Here's the drawing with two shaded views (mm, measured from the low corner). I have some questions. A direction names the side the tool comes from. Coordinates: 2 decimals unless noted, no trailing zeros. Write each loop counter-clockwise with the first axis right and the second up, starting at its lowest first coordinate (ties: lowest second). Pieces come first, ordered by that corner, then holes. Notation, with made-up numbers: (65.25, 66.5) -> (95.25, 66.5) arc R11 cw to (95.25, 71.5) -> close; hole circle Ø8 at (-11, 5). An arc over 180 degrees is marked (long way). Put each result on its own line as item: value.
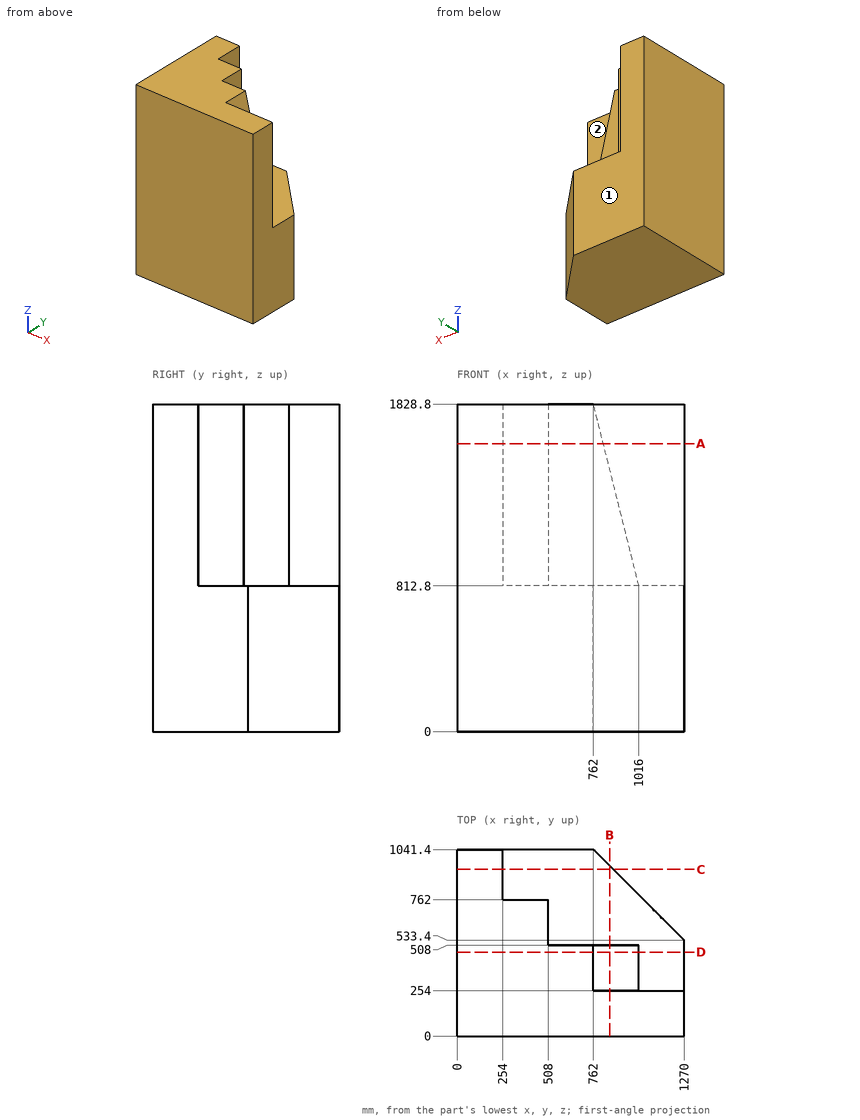
Item 1: Which directions (+Z, -Z, +X, -X, +Y, -Y) give clear straight access to the entire face, cutting with the end or side of a thin tool? Please do the marked faces 1 and 2.
Output:
face 1: +Z, -Z, +X, -X, +Y
face 2: +Z, +X, +Y
Item 2: Imagine slicing it at C-C on y = 930. Write out the boundary of the cut face in (x, z).
Output:
outline: (0, 0) -> (873.4, 0) -> (873.4, 812.8) -> (254, 812.8) -> (254, 1828.8) -> (0, 1828.8) -> close
Item 3: Imagine slicing it at D-D on y = 469. Write out the boundary of the cut face in (x, z), then the cut area to 3 significant figures.
Output:
outline: (0, 0) -> (1270, 0) -> (1270, 812.8) -> (1016, 812.8) -> (762, 1828.8) -> (0, 1828.8) -> close
area: 1,940,000 mm²
Item 4: Please list where these lines run through material, in increasing order: line 1 along X through (y, z) = (530, 1155.5); line 2 along X through (y, z) = (935.5, 972); line 3 along Z through (x, y) = (901, 548). Write a range as from..to.
Output:
line 1: x = 0..508
line 2: x = 0..254
line 3: z = 0..812.8
Item 5: Imagine slicing it at A-A on z = 1608. Write out the boundary of the cut face in (x, y), then the cut area to 3 significant figures.
Output:
outline: (0, 0) -> (1270, 0) -> (1270, 254) -> (817.2, 254) -> (817.2, 508) -> (508, 508) -> (508, 762) -> (254, 762) -> (254, 1041.4) -> (0, 1041.4) -> close
area: 730,000 mm²
Item 6: For P1, Ø12, axis at x = 1042, z = 191.5, coming from the +Y side; P2, Ø12, axis at x = 1078, z = 310.5, coming from the +Y side; P3, Ø12, axis at y = 823.5, z = 1255, coming from the +X side, each with a flat end and sliding along its axis, tell me the tip position at first contact or that it passes through.
Output:
P1: stops at y = 767.4
P2: stops at y = 731.4
P3: stops at x = 254
Item 7: Imagine slicing it at B-B on x = 852.5. Write out the boundary of the cut face in (y, z).
Output:
outline: (0, 0) -> (950.9, 0) -> (950.9, 812.8) -> (508, 812.8) -> (508, 1466.8) -> (254, 1466.8) -> (254, 1828.8) -> (0, 1828.8) -> close
